Geometry check sheet. Reference: the model listing, model coordinates, mm. Face numbers are marked on the shaded views. A direction names the side the tool comes from. Give positions to 0.01 mm unless a question says otherwise; leave off trailing zeros. Order: outer loops, then holes, each group sorted by start corner. A loop starts at its lowest first (then second) coordinate and runs counter-clockwise, first axis right, second up. Notation, with made-up numbers: M 29.5,40.25 L 37.5,40.25 A33 cw 37.5,72.25 Z; hole C 12.5,-10.5 d5. An arc over 180 degrees is marked long. Put each result on its own line as item: value. Start each with the question number.
Q1. Section check A-A on y = 0. Record the cut outline in (x, z), then the cut area to 3 significant figures.
Q2. Access from +Z, -Z, +X, -X, +Y, -Y to the whole of each face (thin tool, end or side, straight path). Record for the marked faces 1, 2, 3 and 4.
Q3. Mould release check, pull along Z, two halves, no side actions. Record for the marked faces 5, 6, 7 and 8: +Z half, -Z half, draft (parallel to the pull), parting line (faces both ways), or undercut.
Q4. Section check D-D on y = 18. Record the cut outline in (x, z).
Q5. Material ranges on L1, parallel to Y at x = 13, z = 1; L2, parallel to X at y = 0, z = 1.6; L3, parallel to Z at x = -17, y = 15.5, recorded low to high.
Q6. Section check C-C on z = -7. Record the cut outline in (x, y), then the cut area to 3 significant figures.
Q7. Section check B-B on x = -18. Record the cut outline in (y, z), then the cut area to 3 significant figures.
Q8. Go/stop test with flat-tipped pins: pin 1 (1.5 mm diameter, centred on x = 4.5, y = 30, fed in from -Z); pin 2 (3 mm diameter, centred on x = -14.5, z = -6, fed in from -Y); pin 3 (2 mm diameter, centred on y = 55.5, z = -8.5, fed in from -X). Record where each tip stops, or that it passes through.
```python
from build123d import *

# Parameters (mm, degrees)
SKETCH_1_W          = 50
SKETCH_1_H          = 20
EXTRUDE_1_DEPTH     = 3
SKETCH_2_W          = 50
SKETCH_2_H          = 12
EXTRUDE_2_DEPTH     = 6
SKETCH_5_W          = 50
SKETCH_5_H          = 9
CUT_EXTRUDE_2_DEPTH = 3
EXTRUDE_3_DEPTH     = 3
EXTRUDE_4_DEPTH     = 55
SKETCH_12_W         = 32.35533906
SKETCH_12_H         = 3
EXTRUDE_6_DEPTH     = 10
EXTRUDE_7_DEPTH     = 3
EXTRUDE_8_DEPTH     = 3
SKETCH_15_R         = 1.65
CUT_EXTRUDE_3_DEPTH = 3


with BuildPart() as part:
    # 草图1 → 凸台-拉伸1 (new body)
    with BuildSketch(Plane.XY):
        Rectangle(SKETCH_1_W, SKETCH_1_H)
        with BuildLine():
            Line((-5.208438024, 2.5), (5.208438024, 2.5))
            ThreePointArc((5.208438024, 2.5), (5.761208823, 2.666666667), (6.129722688, 3.111111111))
            ThreePointArc((6.129722688, 3.111111111), (21.5, 0), (6.129722688, -3.111111111))
            ThreePointArc((6.129722688, -3.111111111), (5.761208823, -2.666666667), (5.208438024, -2.5))
            Line((5.208438024, -2.5), (-5.208438024, -2.5))
            ThreePointArc((-5.208438024, -2.5), (-5.761208823, -2.666666667), (-6.129722688, -3.111111111))
            ThreePointArc((-6.129722688, -3.111111111), (-21.5, 0), (-6.129722688, 3.111111111))
            ThreePointArc((-6.129722688, 3.111111111), (-5.761208823, 2.666666667), (-5.208438024, 2.5))
        make_face(mode=Mode.SUBTRACT)
        with BuildLine():
            Line((3.25, 5.5), (-3.25, 5.5))
            ThreePointArc((-3.25, 5.5), (-5, 7.25), (-3.25, 9))
            Line((-3.25, 9), (3.25, 9))
            ThreePointArc((3.25, 9), (5, 7.25), (3.25, 5.5))
        make_face(mode=Mode.SUBTRACT)
    extrude(amount=EXTRUDE_1_DEPTH)

    # 草图2 → 凸台-拉伸2 (add)
    with BuildSketch(Plane(origin=(0, 10, 0), x_dir=(1, 0, 0), z_dir=(0, 1, 0))):
        with Locations((0, -6)):
            Rectangle(SKETCH_2_W, SKETCH_2_H)
    extrude(amount=EXTRUDE_2_DEPTH)

    # 草图5 → 切除-拉伸2 (cut)
    with BuildSketch(Plane.XZ.offset(-10)):
        with Locations((0, 7.5)):
            Rectangle(SKETCH_5_W, SKETCH_5_H)
    extrude(amount=-CUT_EXTRUDE_2_DEPTH, mode=Mode.SUBTRACT)

    # 草图9 → 凸台-拉伸3 (add)
    with BuildSketch(Plane(origin=(0, 16, 0), x_dir=(1, 0, 0), z_dir=(0, 1, 0))):
        Polygon((25, 0), (0, 25), (-25, 0), align=None)
    extrude(amount=-EXTRUDE_3_DEPTH)

    # 草图11 → 凸台-拉伸4 (add)
    with BuildSketch(Plane(origin=(0, 16, 0), x_dir=(1, 0, 0), z_dir=(0, 1, 0))):
        Polygon((0, 25), (2.121320344, 22.878679656), (-22.878679656, -2.121320344), (-25, 0), align=None)
    extrude(amount=EXTRUDE_4_DEPTH)

    # 草图12 → 凸台-拉伸6 (add)
    with BuildSketch(Plane(origin=(-10.378679656, 0, -10.378679656), x_dir=(0.707106781, 0, -0.707106781), z_dir=(0.707106781, 0, 0.707106781))):
        with Locations((-1.5, 69.5)):
            Rectangle(SKETCH_12_W, SKETCH_12_H)
    extrude(amount=EXTRUDE_6_DEPTH)

    # 草图13 → 凸台-拉伸7 (add)
    with BuildSketch(Plane(origin=(12.5, 0, -12.5), x_dir=(-0.707106781, 0, -0.707106781), z_dir=(0.707106781, 0, -0.707106781))):
        Polygon((14.67766953, 16), (14.67766953, 46), (-0.32233047, 16), align=None)
        Polygon((14.67766953, 46), (14.67766953, 71), (4.67766953, 71), (4.67766953, 68), align=None)
    extrude(amount=-EXTRUDE_7_DEPTH)

    # 草图14 → 凸台-拉伸8 (add)
    with BuildSketch(Plane(origin=(-12.5, 0, 12.5), x_dir=(0.707106781, 0, 0.707106781), z_dir=(-0.707106781, 0, 0.707106781))):
        Polygon((-14.67766953, 46), (-14.67766953, 16), (-4.67766953, 16), align=None)
        Polygon((-14.67766953, 68), (-14.67766953, 46), (-4.67766953, 68), align=None)
    extrude(amount=-EXTRUDE_8_DEPTH)

    # 草图15 → 切除-拉伸3 (cut)
    with BuildSketch(Plane.XZ.offset(-68)):
        with Locations((0.227922061, -13.914213562)):
            Circle(SKETCH_15_R)
        with Locations((-13.914213562, 0.227922061)):
            Circle(SKETCH_15_R)
    extrude(amount=-CUT_EXTRUDE_3_DEPTH, mode=Mode.SUBTRACT)


solid = part.part
```
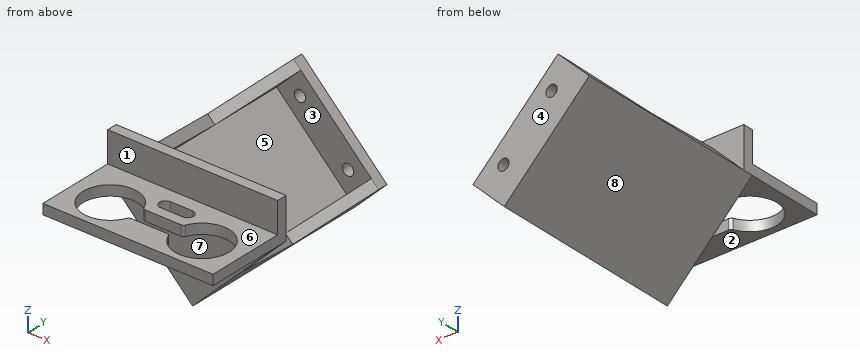
Results found:
1. outline: M -25,0 L -21.5,0 L -21.5,3 L -25,3 Z; M 21.5,0 L 25,0 L 25,3 L 21.5,3 Z
1. area: 21.0 mm^2
2. face 1: +Z, +X, -X, -Y
2. face 2: -Z, +X, -X, -Y
2. face 3: none
2. face 4: +Z, -Z, +X, -X, +Y
3. face 5: undercut
3. face 6: +Z half
3. face 7: draft
3. face 8: -Z half
4. outline: M -25,0 L 0,-25 L 12.02,-12.98 L 9.9,-10.86 L 0,-20.76 L -20.76,0 L -14.16,6.6 L -16.28,8.72 Z
5. L1: y = -10 to -7.98, 7.98 to 16
5. L2: x = -25 to -21.5, 21.5 to 25
5. L3: z = -8 to 12
6. outline: M -18,13 L 18,13 L 18,16 L -13.76,16 L -13.76,68 L 0.38,68 L 0.38,71 L -18,71 Z
6. area: 384 mm^2
7. outline: M -10,0 L -6.61,0 L -6.61,3 L -10,3 Z; M 6.61,0 L 13,0 L 13,-7 L 71,-7 L 71,7 L 61.18,7 L 54.58,2.76 L 68,2.76 L 68,-2.76 L 16,-2.76 L 16,2.76 L 34.3,2.76 L 25.3,7 L 16,7 L 16,12 L 13,12 L 13,3 L 6.61,3 Z
7. area: 450 mm^2
8. pin 1: stops at z = -21.25
8. pin 2: stops at y = 13
8. pin 3: stops at x = -17.5
